from build123d import *

# Parameters (mm, degrees)
SKETCH1_W            = 60
SKETCH1_H            = 60
BOSS_EXTRUDE1_DEPTH  = 10
SKETCH2_R            = 5
CUT_EXTRUDE1_DEPTH   = 11
LPATTERN1_COUNT      = 4
LPATTERN1_PITCH      = 30
LPATTERN1_COUNT_DIR2 = 4
LPATTERN1_PITCH_DIR2 = 30


with BuildPart() as part:
    # Sketch1 → Boss-Extrude1 (new body)
    with BuildSketch(Plane(origin=(0, 0, 0), x_dir=(1, 0, 0), z_dir=(0, 1, 0))):
        with Locations((30, 30)):
            Rectangle(SKETCH1_W, SKETCH1_H)
    extrude(amount=BOSS_EXTRUDE1_DEPTH)

    # Sketch2 → Cut-Extrude1 (cut, through all)
    with BuildSketch(Plane(origin=(0, 10, 0), x_dir=(1, 0, 0), z_dir=(0, 1, 0))):
        with Locations((15, 15)):
            Circle(SKETCH2_R)
    cut_extrude1 = extrude(amount=-CUT_EXTRUDE1_DEPTH, mode=Mode.SUBTRACT)

    # LPattern1: Cut-Extrude1 4 × 4
    with Locations(*[(i * LPATTERN1_PITCH, 0, -j * LPATTERN1_PITCH_DIR2) for i in range(LPATTERN1_COUNT) for j in range(LPATTERN1_COUNT_DIR2) if (i, j) != (0, 0)]):
        add(cut_extrude1, mode=Mode.SUBTRACT)


solid = part.part
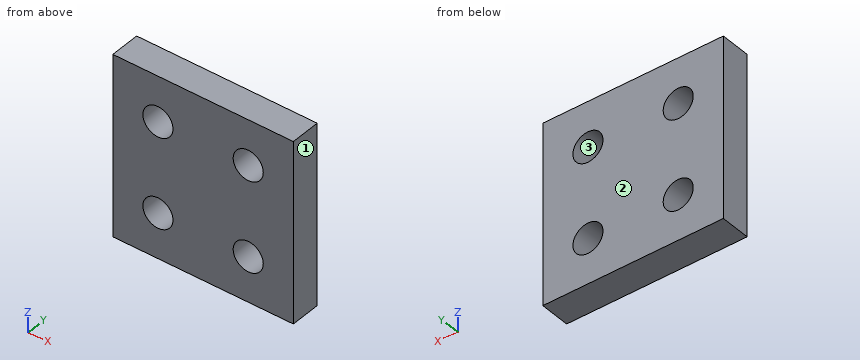
Input: part model. Units: mm. Frame: model coordinates. Face numbers are marked on the shaded views. Give positions to 0.01 mm unless a question says otherwise; leave off trailing zeros. Loops run counter-clockwise (first coordinate to the right, second up) from the corner with the lowest first, then second, coordinate; pieces in that order, holes last. Notation, with made-up numbers: (80, -39.5) - (111, -39.5) arc R20 ccw to (111, -35.5) - close; hole circle Ø9 at (-38.75, 33.5). An arc over 180 degrees is marked (long way). Use CSV: the item, a comma, the result in double quotes. Start each with the question number.
Item 1: Line query: line 1 (X direction, y = 7.5, z = -15); line 2 (Z direction, x = 45, y = 3.25); line 3 (X direction, y = 8.5, z = -47.5). Output: solid intervals per line, ascending.
Item 2: Section B-B on z = -15. Return loops of the section in (x, y).
Item 3: Section A-A on x = 18. Return loops of the section in (y, z).
Item 4: Mould query, pull axis X, two halves, no side actions, for the marked faces 1, 2 and 3. Classes: pulls with the +X half, pulls with the -X half, needs draft (parallel to the pull), parting line crosses it, or undercut.
Item 5: Section C-C on y = 6.75. Return loops of the section in (x, z), then the cut area to 3 significant figures.
Ans:
1,line 1,"x = 0 to 10, 20 to 40, 50 to 60"
1,line 2,"z = -60 to -50, -40 to -20, -10 to 0"
1,line 3,"x = 0 to 10.67, 19.33 to 40.67, 49.33 to 60"
2,outline,"(0, 0) - (10, 0) - (10, 10) - (0, 10) - close; (20, 0) - (40, 0) - (40, 10) - (20, 10) - close; (50, 0) - (60, 0) - (60, 10) - (50, 10) - close"
3,outline,"(0, -60) - (10, -60) - (10, -49) - (0, -49) - close; (0, -41) - (10, -41) - (10, -19) - (0, -19) - close; (0, -11) - (10, -11) - (10, 0) - (0, 0) - close"
4,face 1,"pulls with the +X half"
4,face 2,"needs draft"
4,face 3,"undercut"
5,outline,"(0, -60) - (60, -60) - (60, 0) - (0, 0) - close; hole circle Ø10 at (15, -45); hole circle Ø10 at (15, -15); hole circle Ø10 at (45, -45); hole circle Ø10 at (45, -15)"
5,area,"3,290 mm2"
